Design review of the part built by this model. Coordinates are the model's own, in mm. A direction names the side the tool comes from. Round coordinates to 2 decimals unless told otherwise and drop trailing zeros. Order: outer loops, then holes, each group sorted by start corner. A loop starts at its lowest first (then second) coordinate and runs counter-clockwise, first axis right, second up. Notation, with made-up numbers: (34.25, 73) - (73.25, 73) arc R30 cw to (73.25, 97) - close; hole circle Ø1 at (62.5, 55). An arc over 180 degrees is marked (long way). Use CSV: the item, a comma, the result in double quotes. Start each with the question number.
from build123d import *
from OCP.BRepFilletAPI import BRepFilletAPI_MakeChamfer

# Parameters (mm, degrees)
BOSS_EXTRUDE1_DEPTH = 3.175
CUT_EXTRUDE1_DEPTH  = 0.508
SKETCH3_W           = 21.463
SKETCH3_H           = 16.002
SKETCH3_W_2         = 20.447
SKETCH3_H_2         = 14.986
SKETCH3_W_3         = 15.875
SKETCH3_H_3         = 10.414
CUT_EXTRUDE2_DEPTH  = 2.54
BOSS_EXTRUDE3_DEPTH = 9.906
BOSS_EXTRUDE4_DEPTH = 17.399
SKETCH7_W           = 1.905
SKETCH7_H           = 3.81
CUT_EXTRUDE3_DEPTH  = 16.51
SKETCH8_W           = 1.905
SKETCH8_H           = 3.81
CUT_EXTRUDE4_DEPTH  = 3.81
CHAMFER1_SIZE       = 1.016
CHAMFER1_SIZE2      = 0.586587873
FILLET1_R           = 2.54
SKETCH9_R           = 2.032
CUT_EXTRUDE5_DEPTH  = 44.002957642
CHAMFER2_SIZE       = 1.016
CHAMFER2_SIZE2      = 0.586587873


with BuildPart() as part:
    # Sketch1 → Boss-Extrude1 (new body)
    with BuildSketch(Plane.XY):
        with BuildLine():
            Line((-11.03046671, 29.083), (11.03046671, 29.083))
            ThreePointArc((11.03046671, 29.083), (13.97, 28.146132153), (15.825299343, 25.681088204))
            Line((15.825299343, 25.681088204), (24.225832633, 1.678088204))
            ThreePointArc((24.225832633, 1.678088204), (24.511, 0), (24.225832633, -1.678088204))
            Line((24.225832633, -1.678088204), (15.825299343, -25.681088204))
            ThreePointArc((15.825299343, -25.681088204), (13.97, -28.146132153), (11.03046671, -29.083))
            Line((11.03046671, -29.083), (-11.03046671, -29.083))
            ThreePointArc((-11.03046671, -29.083), (-13.97, -28.146132153), (-15.825299343, -25.681088204))
            Line((-15.825299343, -25.681088204), (-24.225832633, -1.678088204))
            ThreePointArc((-24.225832633, -1.678088204), (-24.511, 0), (-24.225832633, 1.678088204))
            Line((-24.225832633, 1.678088204), (-15.825299343, 25.681088204))
            ThreePointArc((-15.825299343, 25.681088204), (-13.97, 28.146132153), (-11.03046671, 29.083))
        make_face()
    extrude(amount=BOSS_EXTRUDE1_DEPTH)

    # Sketch2 → Cut-Extrude1 (cut)
    with BuildSketch(Plane.XY.offset(3.175)):
        with BuildLine():
            Line((-11.03046671, -29.083), (11.03046671, -29.083))
            ThreePointArc((11.03046671, -29.083), (13.97, -28.146132153), (15.825299343, -25.681088204))
            Line((15.825299343, -25.681088204), (24.225832633, -1.678088204))
            ThreePointArc((24.225832633, -1.678088204), (24.511, 0), (24.225832633, 1.678088204))
            Line((24.225832633, 1.678088204), (15.825299343, 25.681088204))
            ThreePointArc((15.825299343, 25.681088204), (13.97, 28.146132153), (11.03046671, 29.083))
            Line((11.03046671, 29.083), (-11.03046671, 29.083))
            ThreePointArc((-11.03046671, 29.083), (-13.97, 28.146132153), (-15.825299343, 25.681088204))
            Line((-15.825299343, 25.681088204), (-24.225832633, 1.678088204))
            ThreePointArc((-24.225832633, 1.678088204), (-24.511, 0), (-24.225832633, -1.678088204))
            Line((-24.225832633, -1.678088204), (-15.825299343, -25.681088204))
            ThreePointArc((-15.825299343, -25.681088204), (-13.97, -28.146132153), (-11.03046671, -29.083))
        make_face()
        with BuildLine():
            Line((-12.065, 27.305), (12.065, 27.305))
            ThreePointArc((12.065, 27.305), (13.861051224, 26.561051224), (14.605, 24.765))
            Line((14.605, 24.765), (14.605, -24.765))
            ThreePointArc((14.605, -24.765), (13.861051224, -26.561051224), (12.065, -27.305))
            Line((12.065, -27.305), (-12.065, -27.305))
            ThreePointArc((-12.065, -27.305), (-13.861051224, -26.561051224), (-14.605, -24.765))
            Line((-14.605, -24.765), (-14.605, 24.765))
            ThreePointArc((-14.605, 24.765), (-13.861051224, 26.561051224), (-12.065, 27.305))
        make_face(mode=Mode.SUBTRACT)
    extrude(amount=-CUT_EXTRUDE1_DEPTH, mode=Mode.SUBTRACT)

    # Sketch3 → Cut-Extrude2 (cut)
    with BuildSketch(Plane.XY.offset(3.175)):
        with Locations((0, 14.351)):
            Rectangle(SKETCH3_W, SKETCH3_H)
        with Locations((0, 14.351)):
            Rectangle(SKETCH3_W_2, SKETCH3_H_2, mode=Mode.SUBTRACT)
        with Locations((0, 14.351)):
            Rectangle(SKETCH3_W_3, SKETCH3_H_3)
    extrude(amount=-CUT_EXTRUDE2_DEPTH, mode=Mode.SUBTRACT)

    # Sketch5 → Boss-Extrude3 (add)
    with BuildSketch(Plane.XZ.offset(-19.304)):
        with BuildLine():
            Line((-7.6835, 0.635), (-7.6835, 3.175))
            ThreePointArc((-7.6835, 3.175), (-6.408209158, 5.469554889), (-4.313795397, 7.052204524))
            ThreePointArc((-4.313795397, 7.052204524), (-3.908770324, 7.120088215), (-3.527334844, 6.967902539))
            ThreePointArc((-3.527334844, 6.967902539), (1.765964035, 4.148909918), (7.6835, 3.175))
            Line((7.6835, 3.175), (7.6835, 0.635))
            Line((7.6835, 0.635), (-7.6835, 0.635))
        make_face()
    extrude(amount=BOSS_EXTRUDE3_DEPTH)

    # Sketch6 → Boss-Extrude4 (add)
    with BuildSketch(Plane(origin=(0, 0, 0), x_dir=(-1, 0, 0), z_dir=(0, 0, -1))):
        with BuildLine():
            Line((-13.7795, -19.05), (-7.4295, -25.4))
            Line((-7.4295, -25.4), (7.4295, -25.4))
            Line((7.4295, -25.4), (13.7795, -19.05))
            Line((13.7795, -19.05), (13.7795, 19.05))
            ThreePointArc((13.7795, 19.05), (13.035551224, 20.846051224), (11.2395, 21.59))
            Line((11.2395, 21.59), (-11.2395, 21.59))
            ThreePointArc((-11.2395, 21.59), (-13.035551224, 20.846051224), (-13.7795, 19.05))
            Line((-13.7795, 19.05), (-13.7795, -19.05))
        make_face()
    extrude(amount=BOSS_EXTRUDE4_DEPTH)

    # Sketch7 → Cut-Extrude3 (cut)
    with BuildSketch(Plane.XY.offset(3.175)):
        Polygon((-7.3025, -22.352), (7.3025, -22.352), (12.065, -17.5895), (12.065, -5.842), (-12.065, -5.842), (-12.065, -17.5895), align=None)
        with Locations((-8.255, -11.938)):
            Rectangle(SKETCH7_W, SKETCH7_H, mode=Mode.SUBTRACT)
        with Locations((0, -16.256)):
            Rectangle(SKETCH7_W, SKETCH7_H, mode=Mode.SUBTRACT)
        with Locations((8.255, -11.938)):
            Rectangle(SKETCH7_W, SKETCH7_H, mode=Mode.SUBTRACT)
    extrude(amount=-CUT_EXTRUDE3_DEPTH, mode=Mode.SUBTRACT)

    # Sketch8 → Cut-Extrude4 (cut)
    with BuildSketch(Plane.XY.offset(3.175)):
        with Locations((8.255, -11.938)):
            Rectangle(SKETCH8_W, SKETCH8_H)
        with Locations((-8.255, -11.938)):
            Rectangle(SKETCH8_W, SKETCH8_H)
    extrude(amount=-CUT_EXTRUDE4_DEPTH, mode=Mode.SUBTRACT)

    # Chamfer1: one chamfer whose edges measure the first distance from different faces: ONE call of the kernel's chamfer builder (chamfer() names one face for all edges)
    chamfer1_edges_1 = [part.edges().sort_by_distance(p)[0] for p in [
        (-0.9525, -16.256, 3.175),
    ]]
    chamfer1_side_1 = [part.faces().sort_by_distance(p)[0] for p in [
        (-0.9525, -16.256, -5.08),
    ]]
    chamfer1_edges_2 = [part.edges().sort_by_distance(p)[0] for p in [
        (0, -14.351, 3.175),
    ]]
    chamfer1_side_2 = [part.faces().sort_by_distance(p)[0] for p in [
        (0, -14.351, -5.08),
    ]]
    chamfer1_edges_3 = [part.edges().sort_by_distance(p)[0] for p in [
        (0.9525, -16.256, 3.175),
    ]]
    chamfer1_side_3 = [part.faces().sort_by_distance(p)[0] for p in [
        (0.9525, -16.256, -5.08),
    ]]
    chamfer1_edges_4 = [part.edges().sort_by_distance(p)[0] for p in [
        (0, -18.161, 3.175),
    ]]
    chamfer1_side_4 = [part.faces().sort_by_distance(p)[0] for p in [
        (0, -18.161, -5.08),
    ]]
    chamfer1_edges_5 = [part.edges().sort_by_distance(p)[0] for p in [
        (8.255, -10.033, -0.635),
    ]]
    chamfer1_side_5 = [part.faces().sort_by_distance(p)[0] for p in [
        (8.255, -10.033, -6.985),
    ]]
    chamfer1_edges_6 = [part.edges().sort_by_distance(p)[0] for p in [
        (9.2075, -11.938, -0.635),
    ]]
    chamfer1_side_6 = [part.faces().sort_by_distance(p)[0] for p in [
        (9.2075, -11.938, -6.985),
    ]]
    chamfer1_edges_7 = [part.edges().sort_by_distance(p)[0] for p in [
        (8.255, -13.843, -0.635),
    ]]
    chamfer1_side_7 = [part.faces().sort_by_distance(p)[0] for p in [
        (8.255, -13.843, -6.985),
    ]]
    chamfer1_edges_8 = [part.edges().sort_by_distance(p)[0] for p in [
        (7.3025, -11.938, -0.635),
    ]]
    chamfer1_side_8 = [part.faces().sort_by_distance(p)[0] for p in [
        (7.3025, -11.938, -6.985),
    ]]
    chamfer1_edges_9 = [part.edges().sort_by_distance(p)[0] for p in [
        (-8.255, -10.033, -0.635),
    ]]
    chamfer1_side_9 = [part.faces().sort_by_distance(p)[0] for p in [
        (-8.255, -10.033, -6.985),
    ]]
    chamfer1_edges_10 = [part.edges().sort_by_distance(p)[0] for p in [
        (-7.3025, -11.938, -0.635),
    ]]
    chamfer1_side_10 = [part.faces().sort_by_distance(p)[0] for p in [
        (-7.3025, -11.938, -6.985),
    ]]
    chamfer1_edges_11 = [part.edges().sort_by_distance(p)[0] for p in [
        (-8.255, -13.843, -0.635),
    ]]
    chamfer1_side_11 = [part.faces().sort_by_distance(p)[0] for p in [
        (-8.255, -13.843, -6.985),
    ]]
    chamfer1_edges_12 = [part.edges().sort_by_distance(p)[0] for p in [
        (-9.2075, -11.938, -0.635),
    ]]
    chamfer1_side_12 = [part.faces().sort_by_distance(p)[0] for p in [
        (-9.2075, -11.938, -6.985),
    ]]
    chamfer1 = BRepFilletAPI_MakeChamfer(part.part.solid().wrapped)
    for e in chamfer1_edges_1:
        chamfer1.Add(CHAMFER1_SIZE, CHAMFER1_SIZE2, e.wrapped, chamfer1_side_1[0].wrapped)  # the first distance lies on this face
    for e in chamfer1_edges_2:
        chamfer1.Add(CHAMFER1_SIZE, CHAMFER1_SIZE2, e.wrapped, chamfer1_side_2[0].wrapped)  # the first distance lies on this face
    for e in chamfer1_edges_3:
        chamfer1.Add(CHAMFER1_SIZE, CHAMFER1_SIZE2, e.wrapped, chamfer1_side_3[0].wrapped)  # the first distance lies on this face
    for e in chamfer1_edges_4:
        chamfer1.Add(CHAMFER1_SIZE, CHAMFER1_SIZE2, e.wrapped, chamfer1_side_4[0].wrapped)  # the first distance lies on this face
    for e in chamfer1_edges_5:
        chamfer1.Add(CHAMFER1_SIZE, CHAMFER1_SIZE2, e.wrapped, chamfer1_side_5[0].wrapped)  # the first distance lies on this face
    for e in chamfer1_edges_6:
        chamfer1.Add(CHAMFER1_SIZE, CHAMFER1_SIZE2, e.wrapped, chamfer1_side_6[0].wrapped)  # the first distance lies on this face
    for e in chamfer1_edges_7:
        chamfer1.Add(CHAMFER1_SIZE, CHAMFER1_SIZE2, e.wrapped, chamfer1_side_7[0].wrapped)  # the first distance lies on this face
    for e in chamfer1_edges_8:
        chamfer1.Add(CHAMFER1_SIZE, CHAMFER1_SIZE2, e.wrapped, chamfer1_side_8[0].wrapped)  # the first distance lies on this face
    for e in chamfer1_edges_9:
        chamfer1.Add(CHAMFER1_SIZE, CHAMFER1_SIZE2, e.wrapped, chamfer1_side_9[0].wrapped)  # the first distance lies on this face
    for e in chamfer1_edges_10:
        chamfer1.Add(CHAMFER1_SIZE, CHAMFER1_SIZE2, e.wrapped, chamfer1_side_10[0].wrapped)  # the first distance lies on this face
    for e in chamfer1_edges_11:
        chamfer1.Add(CHAMFER1_SIZE, CHAMFER1_SIZE2, e.wrapped, chamfer1_side_11[0].wrapped)  # the first distance lies on this face
    for e in chamfer1_edges_12:
        chamfer1.Add(CHAMFER1_SIZE, CHAMFER1_SIZE2, e.wrapped, chamfer1_side_12[0].wrapped)  # the first distance lies on this face
    add(Compound.cast(chamfer1.Shape()), mode=Mode.REPLACE)

    # Fillet1
    fillet1_edges = [part.edges().sort_by_distance(p)[0] for p in [
        (-12.065, -5.842, -5.08),
        (12.065, -5.842, -5.08),
    ]]
    fillet(fillet1_edges, radius=FILLET1_R)

    # Sketch9 → Cut-Extrude5 (cut, through all)
    with BuildSketch(Plane.XY.offset(2.667)):
        with Locations((-19.431, 0)):
            Circle(SKETCH9_R)
        with Locations((19.431, 0)):
            Circle(SKETCH9_R)
    extrude(amount=-CUT_EXTRUDE5_DEPTH, mode=Mode.SUBTRACT)

    # Chamfer2
    chamfer2_edges = [part.edges().sort_by_distance(p)[0] for p in [
        (-21.463, 0, 2.667),
        (17.399, 0, 2.667),
    ]]
    chamfer2_side = [part.faces().sort_by_distance(p)[0] for p in [
        (-23.750313465, 0, 2.667),
    ]]
    chamfer(chamfer2_edges, length=CHAMFER2_SIZE, length2=CHAMFER2_SIZE2, reference=chamfer2_side[0])


solid = part.part
Q1. Tool access review of faces 5 (the flat face through (0, -18.161, -5)), 6 (the flat face through (0, 21.59, -9)), 7 (the cylindrical face through (-13.88, 26.54, 2.92)): name each direction out of +Z, -Z, +X, -X, +Y, -Y from which nothing blocks a thin tool from reaching the whole face with its end or side.
Q2. Clearance check with flat-ended pins moving along their axes: pin 1 (12 mm diameter, centred on x = 14, z = -11, fed in from -Y); pin 2 (10 mm diameter, centred on x = -6.5, y = -18, fed in from +Z) (3 decimals); pin 3 (0.6 mm diameter, centred on y = 5, z = 3, fed in from +X) (3 decimals); pin 4 (10 mm diameter, centred on x = 3, z = 3.5, fed in from -Y). State where each tip first meets the part, or that it passes through.
Q3. For L1, parallel to Y at x = 0.5, z = -5.75; L2, parallel to Y at x = 6, z = -2.75; L3, parallel to Y at x = -9, z = -13, list the stretches that pass through material, from the lowest coordinate up. Write a range as [from, to].
Q4. Take a section at A-A (z = -10.25). Give the number of separate pieces and of enclosed holes in the cut face, plus the area to 3 significant figures.
Q5. Take a section at C-C (z = -15.5). State the section outline as (x, y) points, plus the area to 3 significant figures.
Q6. The part is to be moulded in two halves that separate along X. For faces 1 (the flat face through (0, 6.35, 2)), 2 (the flat face through (0, 8, 3.175)), 3 (the flat face through (7.303, -12, -7)), 4 (the cylindrical face through (-14.006, 28.121, 1.315)), say which applies: +X half, -X half, draft (parallel to the pull), parting line (faces both ways), or undercut.
Q7. Take a section at B-B (y = 0). State the section outline as (x, z) points (1 decimal), plus the area to 3 significant figures.
Findings below:
1,face 5,"+Z"
1,face 6,"-Z, +X, -X, +Y"
1,face 7,"+Z, -X, +Y"
2,pin 1,"stops at y = -24.83"
2,pin 2,"stops at z = 3.175"
2,pin 3,"stops at x = 14.605"
2,pin 4,"stops at y = -29.08"
3,L1,"y = [-25.4, -22.35], [-18.16, -14.35], [-5.84, 21.59]"
3,L2,"y = [-25.4, -22.35], [-5.84, 21.59]"
3,L3,"y = [-23.83, -20.65], [-13.84, -10.03], [-5.84, 21.59]"
4,separate pieces,"4"
4,enclosed holes,"1"
4,area,"901 mm^2"
5,outline,"(-13.78, -19.05) - (-7.43, -25.4) - (7.43, -25.4) - (13.78, -19.05) - (13.78, 19.05) arc R2.54 ccw to (11.24, 21.59) - (-11.24, 21.59) arc R2.54 ccw to (-13.78, 19.05) - close"
5,area,"1,250 mm^2"
6,face 1,"undercut"
6,face 2,"draft"
6,face 3,"undercut"
6,face 4,"-X half"
7,outline,"(-24.5, 0) - (-21.5, 0) - (-21.5, 2.1) - (-22.5, 2.7) - (-24.5, 2.7) - close; (-17.4, 0) - (-13.8, 0) - (-13.8, -17.4) - (13.8, -17.4) - (13.8, 0) - (17.4, 0) - (17.4, 2.1) - (16.4, 2.7) - (14.6, 2.7) - (14.6, 3.2) - (-14.6, 3.2) - (-14.6, 2.7) - (-16.4, 2.7) - (-17.4, 2.1) - close; (21.5, 0) - (24.5, 0) - (24.5, 2.7) - (22.5, 2.7) - (21.5, 2.1) - close"
7,area,"602 mm^2"
